Part model, mm, in its own coordinate system. Face numbers are marked on the shaded views. A direction names the side the tool comes from. Round coordinates to 2 decimals unless told otherwise and drop trailing zeros. Write each loop counter-clockwise with the first axis right and the second up, starting at its lowest first coordinate (ties: lowest second). Pieces come first, ordered by that corner, then holes. Notation, with made-up numbers: (42.5, -35.5) -> (80.5, -35.5) arc R21 ccw to (80.5, -23.5) -> close; hole circle Ø2 at (80.25, 32). An arc over 180 degrees is marked (long way). Use CSV: the item, a comma, the result in double quotes. Start each with the question number.
(1) Saw through at A-A (x = -8.5). Give the cut face in (y, z).
(2) Drop flat-ended pins along their axis: pin 1 (2 mm diameter, centred on y = -0.5, z = -2, fed in from +X); pin 2 (1 mm diameter, centred on x = -5, y = 0, fed in from -Z); pin 3 (2 mm diameter, centred on x = -8.5, y = 0.5, fed in from +Z); pin 4 (1.2 mm diameter, centred on x = -15, y = -0.5, fed in from -Z). Give the stop position or say it passes through.
(3) Probe line 1 (X direction, y = 0.75, z = -1); line 2 (X direction, y = -1.75, z = 4); line 3 (Y direction, x = -1.75, z = -1.75). List the from-to ranges inside material, lowest first. Write a range as [from, to].
(4) Which spindle directions (+Z, -Z, +X, -X, +Y, -Y) get a long thin tool onto all of the face, cutting with end or side? Do the marked faces 4 and 5. Say none if no direction does.
(5) Two-plate mould, pull along Y, no slides. Class the marked faces 1, 2 and 3: released by +Y, released by -Y, zero draft, split by the parting line, or undercut.
```python
from build123d import *

# Parameters (mm, degrees)
CUT_EXTRUDE_1_DEPTH = 2.58


with BuildPart() as part:
    # Sketch 1 → Revolve 1 (revolve)
    with BuildSketch(Plane.XY):
        with BuildLine():
            Line((0, 2), (-13.435105037, 2))
            ThreePointArc((-13.435105037, 2), (-13.513251262, 2.015899029), (-13.578972997, 2.061068326))
            Line((-13.578972997, 2.061068326), (-15.914908162, 4.48))
            Line((-15.914908162, 4.48), (-16, 4.48))
            Line((-16, 4.48), (-16, 0))
            Line((-16, 0), (0, 0))
            Line((0, 0), (0, 2))
        make_face()
    revolve(axis=Axis((0, 0, 0), (-1, 0, 0)))

    # Sketch 2 → Cut-Extrude 1 (cut)
    with BuildSketch(Plane.ZY.offset(16)):
        Polygon((0, 1.443375673), (-1.25, 0.721687836), (-1.25, -0.721687836), (0, -1.443375673), (1.25, -0.721687836), (1.25, 0.721687836), align=None)
    extrude(amount=-CUT_EXTRUDE_1_DEPTH, mode=Mode.SUBTRACT)

    # Sketch 6 → Revolve 2 (revolve)
    with BuildSketch(Plane.XY):
        Polygon((-14.5, 1.443375673), (-13.666666667, 0), (-13.05, 0), (-13.05, 1.443375673), align=None)
    revolve(axis=Axis((-16, 0, 0), (1, 0, 0)))

    # Sketch 7 → Cut-Revolve 2 (revolve, cut)
    with BuildSketch(Plane.XY):
        Polygon((-16, 1.443375673), (-16, 0), (-15.593, 0), align=None)
    revolve(axis=Axis((-16, 0, 0), (1, 0, 0)), mode=Mode.SUBTRACT)

    # Sketch 4 → Cut-Revolve 1 (revolve, cut)
    with BuildSketch(Plane.XY):
        Polygon((-0.35, 2), (0, 1.393782217), (0.35, 2), align=None)
    revolve(axis=Axis((-0.35, 0, 0), (1, 0, 0)), mode=Mode.SUBTRACT)


solid = part.part
```
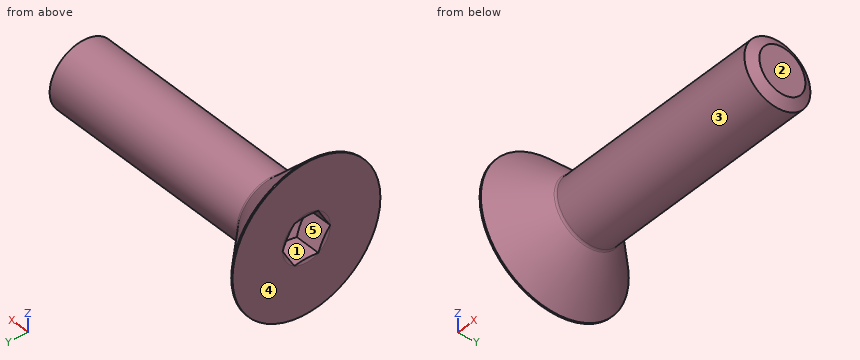
Answers:
1,outline,"circle Ø4 at (0, 0)"
2,pin 1,"stops at x = 0"
2,pin 2,"stops at z = -2"
2,pin 3,"stops at z = 2"
2,pin 4,"stops at z = -4.13"
3,line 1,"x = [-14.39, 0]"
3,line 2,"x = [-16, -15.8]"
3,line 3,"y = [-0.97, 0.97]"
4,face 4,"+Z, -Z, -X, +Y, -Y"
4,face 5,"-X"
5,face 1,"undercut"
5,face 2,"zero draft"
5,face 3,"split by the parting line"
